```python
from build123d import *

# Parameters (mm, degrees)
SKETCH2_R          = 1.046208244
CUT_EXTRUDE1_DEPTH = 4
SKETCH3_R          = 1
CUT_EXTRUDE2_DEPTH = 3


with BuildPart() as part:
    # Sketch1 → Revolve1 (revolve)
    with BuildSketch(Plane.XY, mode=Mode.PRIVATE) as revolve1_sk:
        Polygon((0, 23.312815917), (0, 0), (0, -22.187184083), (10.054416675, -22.187184083), (18, -22.187184083), (20, -20.187184083), (20, -19.187184083), (19.5, -19.187184083), (19.5, -18.687184083), (20, -18.687184083), (20, -17.687184083), (18, -17.687184083), (18, -17.387184083), (20, -17.387184083), (20, 14.312815917), (16, 18.312815917), (2, 18.312815917), (2, 23.312815917), align=None)
        Polygon((2, 17.312815917), (15.585786438, 17.312815917), (19, 13.898602354), (19, 12.898602354), (1, 12.898602354), (1, 16.312815917), (2, 16.312815917), align=None, mode=Mode.SUBTRACT)
    revolve(revolve1_sk.sketch.rotate(Axis((0, 23.312815917, 0), (0, -1, 0)), 180), axis=Axis((0, 23.312815917, 0), (0, -1, 0)))

    # Sketch2 → Cut-Extrude1 (cut)
    with BuildSketch(Plane(origin=(0, 18.312815917, 0), x_dir=(1, 0, 0), z_dir=(0, 1, 0))):
        with Locations(Location((0, -5.211771178, 0), (0, 0, 270))):
            Circle(SKETCH2_R)
        with Locations(Location((-5.211771178, 0, 0), (0, 0, 270))):
            Circle(SKETCH2_R)
        with Locations(Location((0, 5.211771178, 0), (0, 0, 270))):
            Circle(SKETCH2_R)
        with Locations(Location((5.211771178, 0, 0), (0, 0, 270))):
            Circle(SKETCH2_R)
        with BuildLine():
            Line((-3, 9.577417814), (-3, 16.838236804))
            Line((-3, 16.838236804), (3, 16.838236804))
            Line((3, 16.838236804), (3, 9.577417814))
            ThreePointArc((3, 9.577417814), (0, 6.577417814), (-3, 9.577417814))
        make_face()
        with BuildLine():
            Line((16.082340827, 5.821042191), (9.794287129, 2.190632695))
            ThreePointArc((9.794287129, 2.190632695), (5.696210918, 3.288708907), (6.794287129, 7.386785118))
            Line((6.794287129, 7.386785118), (13.082340827, 11.017194613))
            Line((13.082340827, 11.017194613), (16.082340827, 5.821042191))
        make_face()
        with BuildLine():
            Line((13.082340827, -11.017194613), (6.794287129, -7.386785118))
            ThreePointArc((6.794287129, -7.386785118), (5.696210918, -3.288708907), (9.794287129, -2.190632695))
            Line((9.794287129, -2.190632695), (16.082340827, -5.821042191))
            Line((16.082340827, -5.821042191), (13.082340827, -11.017194613))
        make_face()
        with BuildLine():
            Line((-3, -16.838236804), (-3, -9.577417814))
            ThreePointArc((-3, -9.577417814), (0, -6.577417814), (3, -9.577417814))
            Line((3, -9.577417814), (3, -16.838236804))
            Line((3, -16.838236804), (-3, -16.838236804))
        make_face()
        with BuildLine():
            Line((-16.082340827, -5.821042191), (-9.794287129, -2.190632695))
            ThreePointArc((-9.794287129, -2.190632695), (-5.696210918, -3.288708907), (-6.794287129, -7.386785118))
            Line((-6.794287129, -7.386785118), (-13.082340827, -11.017194613))
            Line((-13.082340827, -11.017194613), (-16.082340827, -5.821042191))
        make_face()
        with BuildLine():
            Line((-13.082340827, 11.017194613), (-6.794287129, 7.386785118))
            ThreePointArc((-6.794287129, 7.386785118), (-5.696210918, 3.288708907), (-9.794287129, 2.190632695))
            Line((-9.794287129, 2.190632695), (-16.082340827, 5.821042191))
            Line((-16.082340827, 5.821042191), (-13.082340827, 11.017194613))
        make_face()
    extrude(amount=-CUT_EXTRUDE1_DEPTH, mode=Mode.SUBTRACT)

    # Sketch3 → Cut-Extrude2 (cut)
    with BuildSketch(Plane.XZ.offset(22.187184083)):
        with Locations(Location((0, -9.5, 0), (0, 0, 270))):
            Circle(SKETCH3_R)
        with Locations(Location((-12.5, 0, 0), (0, 0, 270))):
            Circle(SKETCH3_R)
        with Locations(Location((0, 9.5, 0), (0, 0, 270))):
            Circle(SKETCH3_R)
        with Locations(Location((12.5, 0, 0), (0, 0, 270))):
            Circle(SKETCH3_R)
    extrude(amount=-CUT_EXTRUDE2_DEPTH, mode=Mode.SUBTRACT)


solid = part.part
```
The model under review builds one solid part; all positions refer to its coordinate system, in mm. A direction names the side the tool comes from. Round coordinates to 2 decimals unless told otherwise and drop trailing zeros. Loops run counter-clockwise (first coordinate to the right, second up) from the corner with the lowest first, then second, coordinate; pieces in that order, holes last. Notation, with made-up numbers: (86, 62) -> (103, 62) arc R35 cw to (103, 98) -> close; hole circle Ø5 at (-7, -11.75). An arc over 180 degrees is marked (long way). Answer as a JSON object with one key per item and string values. Group by question number.
1) We need section A-A on y = -11.5. Write out the cut boundary in (x, z).
2) For faces 4 (the face through (4.119, 13.392, 18.548)), 5 (the face through (-0.6, -20.7, -8.7)), 6 (the face through (19.98, -1.32, -0.88)), 7 (the face through (12.98, 17.63, -4.03)), list the 3-axis set-ups (+Z, -Z, +X, -X, +Y, -Y) from which the entire face can be reached by the end or side of a thin tool; tool diameter is ignored.
3) We need section B-B on x = 0. Give the number of separate pieces and of enclosed holes in the cut face, then the cut area to 3 significant figures.
4) Mouldability with a two-part tool opening along Y and no side actions: class faces 1 (the face through (-6.233, 17.82, -0.227)), 2 (the face through (3.51, 18.12, 15.81)), 3 (the face through (0, 12.899, 4)) as released by +Y, released by -Y, zero draft, split by the parting line, or undercut.
5) We need section C-C on y = 20.5. Write out the cut boundary in (x, z), then the cut area to 3 significant figures.
6) For pin 1 Ø0.6 at (x, z) = (-12.5, 0.5) entering from -Y; pin 2 Ø1.3 at (x, y) = (1, 16.5) entering from -Z; pin 3 Ø2 at (y, z) = (17, 13.5) entering from +X; pin 4 Ø2.5 at (x, z) = (-12.5, 0) entering from -Y, all flat-tipped, find the tip position at first contact; note any pin that passes through.
7) For line 1 (Z direction, x = 0, y = 13.75); line 2 (Y direction, x = 4.5, z = -17.5); line 3 (Y direction, x = 14.5, z = 12), list the stretches that pass through material, from the lowest coordinate up. Write a range as [from, to].
Result set:
{
 "1": {"outline": "circle Ø40 at (0, 0)"},
 "2": {"face 4": "none", "face 5": "-Y", "face 6": "+Y, -Y", "face 7": "+Y"},
 "3": {"separate pieces": "3", "enclosed holes": "0", "area": "1,440 mm²"},
 "4": {"face 1": "zero draft", "face 2": "released by +Y", "face 3": "undercut"},
 "5": {"outline": "circle Ø4 at (0, 0)", "area": "12.6 mm²"},
 "6": {"pin 1": "y = -19.19", "pin 2": "z = -18.44", "pin 3": "x = 12.72", "pin 4": "y = -22.19"},
 "7": {"line 1": "[-20, -19], [-1, 1], [19, 20]", "line 2": "[-22.12, -17.69], [-17.39, 12.9], [14.83, 16.24]", "line 3": "[-21.37, -17.69], [-17.39, 12.9], [14.08, 15.49]"}
}
